Verification items for this drawing (mm, ordinates from the low corner). Coordinates: 2 decimals unless noted, no trailing zeros. Write each loop counter-clockwise with the first axis right and the second up, starting at its lowest first coordinate (ties: lowest second). Pieces come first, ordered by that corner, then holes.
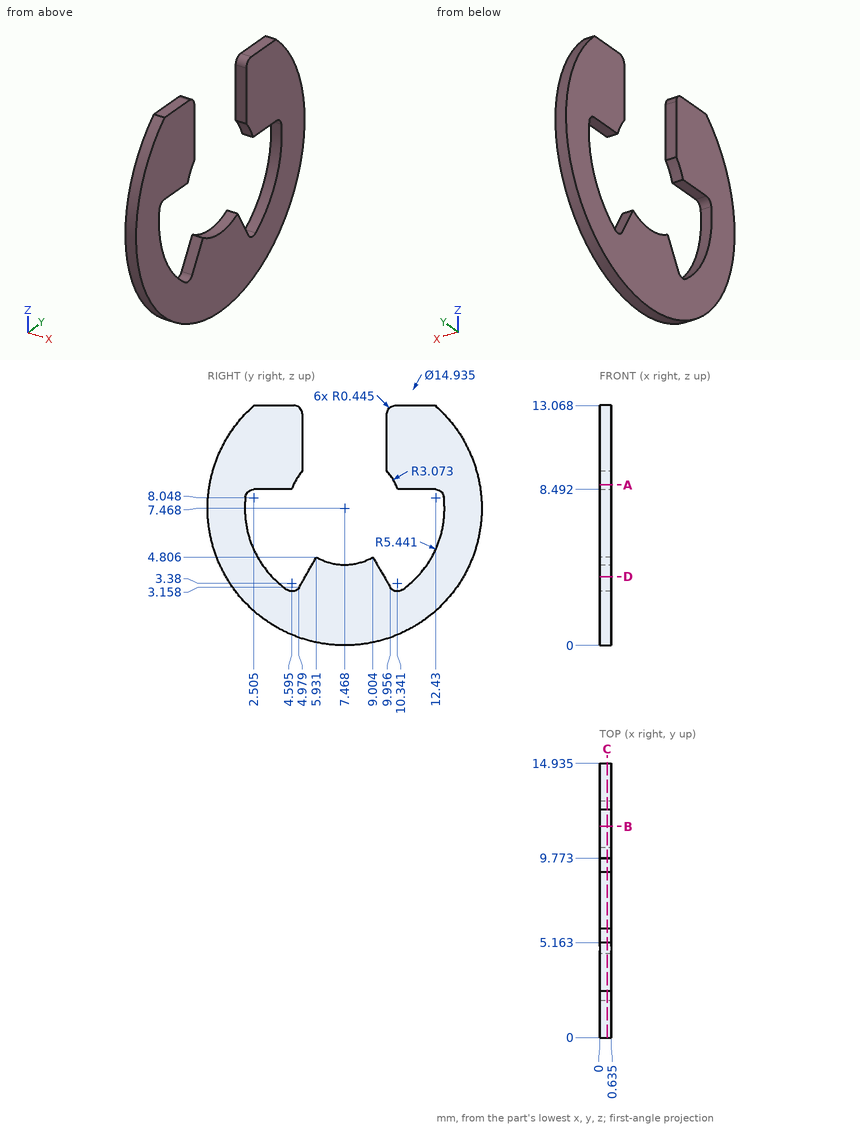
1. Thickness scan on line 1 along Y through (x, z) = (0.25, 7.25); line 2 along Z through (x, y) = (0.5, 12.25) (1 decimal); line 3 along Y through (x, z) = (0.5, 5) (1 decimal). Record the ranges inside material, lowest first.
Computed values:
line 1: y = 0 to 2.03, 12.9 to 14.93
line 2: z = 1.7 to 4.9, 8.5 to 13.1
line 3: y = 0.4 to 2.6, 12.3 to 14.5
2. Sectioned sample at C-C, the plane x = 0.4. Record the boundary of the cut face in (y, z) (1 decimal).
Computed values:
outline: (2.1, 8.1) arc R0.4 cw to (2.5, 8.5) - (4.6, 8.5) arc R3.1 cw to (5.2, 9.5) - (5.2, 12.6) arc R0.4 ccw to (4.7, 13.1) - (2.5, 13.1) arc R7.5 ccw (long way) to (12.4, 13.1) - (10.2, 13.1) arc R0.4 ccw to (9.8, 12.6) - (9.8, 9.5) arc R3.1 cw to (10.4, 8.5) - (12.4, 8.5) arc R0.4 cw to (12.9, 8.1) arc R5.4 cw to (10.6, 3) arc R0.4 cw to (10, 3.2) - (9, 4.8) arc R3.1 cw to (5.9, 4.8) - (5, 3.2) arc R0.4 cw to (4.3, 3) arc R5.4 cw to start
3. Sectioned sample at A-A, the plane z = 8.75. Record the boundary of the cut face in (x, y) (1 decimal).
Computed values:
outline: (0, 0.1) - (0.6, 0.1) - (0.6, 4.7) - (0, 4.7) - close; (0, 10.3) - (0.6, 10.3) - (0.6, 14.8) - (0, 14.8) - close
4. Sectioned sample at D-D, the plane z = 3.75. Record the boundary of the cut face in (x, y) (1 decimal).
Computed values:
outline: (0, 1) - (0.6, 1) - (0.6, 3.5) - (0, 3.5) - close; (0, 5.3) - (0.6, 5.3) - (0.6, 9.6) - (0, 9.6) - close; (0, 11.4) - (0.6, 11.4) - (0.6, 13.9) - (0, 13.9) - close
5. Sectioned sample at B-B, the plane y = 11.5. Record the boundary of the cut face in (x, z) (1 decimal).
Computed values:
outline: (0, 1.2) - (0.6, 1.2) - (0.6, 3.8) - (0, 3.8) - close; (0, 8.5) - (0.6, 8.5) - (0.6, 13.1) - (0, 13.1) - close
